Read the model definition and answer for the solid it produces. Units are mm, in the model's axes. A direction names the side the tool comes from. Round coordinates to 2 decimals unless told otherwise and drop trailing zeros. Order: outer loops, then holes, each group sorted by start corner. A loop starts at its lowest first (then second) coordinate and runs counter-clockwise, first axis right, second up. Notation, with made-up numbers: (60.25, -24) -> (114.25, -24) arc R20 cw to (114.25, 13) -> close; hole circle Ø1 at (19, 77). An arc over 180 degrees is marked (long way). Use a Markdown table: item, result. Add a question column.
1. Section A-A, the plane z = 48.5 is taken. Give the vertices of the cut face in (x, y), then the cut area to 3 significant figures.
2. For faces 1 (the face through (-66, 3, 78)), 2 (the face through (42, 3, -105)), 3 (the face through (62.5, 3, -96)), 4 (the face through (65, 3, 66)), determine the directions among +Z, -Z, +X, -X, +Y, -Y from which every point of the face is accessible in a straight line to the end or side of a thin tool.
3. Given pin 1 (3 mm diameter, centred on x = -17.5, y = 4, fed in from -Z); pin 2 (3 mm diameter, centred on x = -66, y = 3, fed in from +Z); pin 3 (3 mm diameter, centred on y = 4, z = -99, fed in from -X); pin 4 (1.8 mm diameter, centred on y = 3, z = -105, fed in from +X), each flat-ended and moving along its own axis, determine where each tip first touches the part or whether it passes through.
4. The mould has two halves that part along X. Classify faces 5 (the face through (-66, 3, 42)), 6 (the face through (-42, 3, -105)), 7 (the face through (68.5, 3, -84)), 8 (the face through (-68.5, 3, 60)): +X half, -X half, draft (parallel to the pull), parting line (faces both ways), or undercut.
5. Consider L1, parallel to X at y = 2.4, z = 48.5; L2, parallel to Z at x = 10, y = 3.75; L3, parallel to X at y = 2.2, z = 70. Determine where each line is inside the solid, lowest interval first. Write a range as [from, to].
```python
from build123d import *

# Parameters (mm, degrees)
SKETCH3_W           = 125
SKETCH3_H           = 205
BOSS_EXTRUDE1_DEPTH = 6
SKETCH5_W           = 12
SKETCH5_H           = 6
SKETCH5_W_2         = 6
SKETCH5_H_2         = 12
BOSS_EXTRUDE2_DEPTH = 6
SKETCH6_R           = 10
CUT_EXTRUDE1_DEPTH  = 6


with BuildPart() as part:
    # Sketch3 → Boss-Extrude1 (new body)
    with BuildSketch(Plane(origin=(0, 0, 0), x_dir=(1, 0, 0), z_dir=(0, 1, 0))):
        Rectangle(SKETCH3_W, SKETCH3_H)
    extrude(amount=BOSS_EXTRUDE1_DEPTH)

    # Sketch5 → Boss-Extrude2 (add)
    with BuildSketch(Plane(origin=(0, 6, 0), x_dir=(1, 0, 0), z_dir=(0, 1, 0))):
        with Locations((24, -105.5)):
            Rectangle(SKETCH5_W, SKETCH5_H)
        with Locations((0, -105.5)):
            Rectangle(SKETCH5_W, SKETCH5_H)
        with Locations((-65.5, -84)):
            Rectangle(SKETCH5_W_2, SKETCH5_H_2)
        with Locations((-65.5, -60)):
            Rectangle(SKETCH5_W_2, SKETCH5_H_2)
        with Locations((-65.5, -12)):
            Rectangle(SKETCH5_W_2, SKETCH5_H_2)
        with Locations((65.5, -84)):
            Rectangle(SKETCH5_W_2, SKETCH5_H_2)
        with Locations((65.5, -36)):
            Rectangle(SKETCH5_W_2, SKETCH5_H_2)
        with Locations((65.5, -12)):
            Rectangle(SKETCH5_W_2, SKETCH5_H_2)
        with Locations((65.5, 12)):
            Rectangle(SKETCH5_W_2, SKETCH5_H_2)
        with Locations((65.5, 36)):
            Rectangle(SKETCH5_W_2, SKETCH5_H_2)
        with Locations((65.5, 84)):
            Rectangle(SKETCH5_W_2, SKETCH5_H_2)
        with Locations((24, 105.5)):
            Rectangle(SKETCH5_W, SKETCH5_H)
        with Locations((0, 105.5)):
            Rectangle(SKETCH5_W, SKETCH5_H)
        with Locations((-24, 105.5)):
            Rectangle(SKETCH5_W, SKETCH5_H)
        with Locations((-48, 105.5)):
            Rectangle(SKETCH5_W, SKETCH5_H)
        with Locations((-65.5, 36)):
            Rectangle(SKETCH5_W_2, SKETCH5_H_2)
        with Locations((-65.5, 12)):
            Rectangle(SKETCH5_W_2, SKETCH5_H_2)
        with Locations((48, -105.5)):
            Rectangle(SKETCH5_W, SKETCH5_H)
        with Locations((-24, -105.5)):
            Rectangle(SKETCH5_W, SKETCH5_H)
        with Locations((-48, -105.5)):
            Rectangle(SKETCH5_W, SKETCH5_H)
        with Locations((-65.5, -36)):
            Rectangle(SKETCH5_W_2, SKETCH5_H_2)
        with Locations((65.5, -60)):
            Rectangle(SKETCH5_W_2, SKETCH5_H_2)
        with Locations((65.5, 60)):
            Rectangle(SKETCH5_W_2, SKETCH5_H_2)
        with Locations((48, 105.5)):
            Rectangle(SKETCH5_W, SKETCH5_H)
        with Locations((-65.5, 84)):
            Rectangle(SKETCH5_W_2, SKETCH5_H_2)
        with Locations((-65.5, 60)):
            Rectangle(SKETCH5_W_2, SKETCH5_H_2)
    extrude(amount=-BOSS_EXTRUDE2_DEPTH)

    # Sketch6 → Cut-Extrude1 (cut)
    with BuildSketch(Plane(origin=(0, 6, 0), x_dir=(1, 0, 0), z_dir=(0, 1, 0))):
        with Locations((22.512507822, -48.5)):
            Circle(SKETCH6_R)
    extrude(amount=-CUT_EXTRUDE1_DEPTH, mode=Mode.SUBTRACT)


solid = part.part
```
Verdict:
| question | item | result |
|---|---|---|
| 1 | outline | (-62.5, 0) -> (12.51, 0) -> (12.51, 6) -> (-62.5, 6) -> close; (32.51, 0) -> (62.5, 0) -> (62.5, 6) -> (32.51, 6) -> close |
| 1 | area | 630 mm2 |
| 2 | face 1 | -X, +Y, -Y |
| 2 | face 2 | -Z, +Y, -Y |
| 2 | face 3 | -Z, +X, +Y, -Y |
| 2 | face 4 | +X, +Y, -Y |
| 3 | pin 1 | stops at z = -108.5 |
| 3 | pin 2 | stops at z = 90 |
| 3 | pin 3 | stops at x = -62.5 |
| 3 | pin 4 | stops at x = 54 |
| 4 | face 5 | draft |
| 4 | face 6 | undercut |
| 4 | face 7 | +X half |
| 4 | face 8 | -X half |
| 5 | L1 | x = [-62.5, 12.51], [32.51, 62.5] |
| 5 | L2 | z = [-102.5, 102.5] |
| 5 | L3 | x = [-62.5, 62.5] |
